```python
from build123d import *

# Parameters (mm, degrees)
F0_R     = 20.2565
F0_R_2   = 1.5875
F1_DEPTH = 1.27


with BuildPart() as f1:
    # F0 (on Top) → F1 (new body)
    with BuildSketch(Plane.XY):
        Circle(F0_R)
        with Locations((-11.1125, -11.1125)):
            Circle(F0_R_2, mode=Mode.SUBTRACT)
        with Locations((11.1125, -11.1125)):
            Circle(F0_R_2, mode=Mode.SUBTRACT)
        with Locations((-11.1125, 11.1125)):
            Circle(F0_R_2, mode=Mode.SUBTRACT)
        with BuildLine():
            ThreePointArc((0.317454, 9.341808), (6.720768, 6.496262), (9.3472, 0))
            ThreePointArc((9.3472, 0), (-6.496262, -6.720768), (-0.317454, 9.341808))
            ThreePointArc((-0.317454, 9.341808), (-0.002696, 9.664689), (0.3175, 9.3472))
            ThreePointArc((0.3175, 9.3472), (0.317489, 9.344504), (0.317454, 9.341808))
        make_face(mode=Mode.SUBTRACT)
        with Locations((11.1125, 11.1125)):
            Circle(F0_R_2, mode=Mode.SUBTRACT)
    extrude(amount=F1_DEPTH)


solid = f1.part
```
Read the model definition and answer for the solid it produces. Units are mm, in the model's axes. Coordinates: 2 decimals unless noted, no trailing zeros. Order: outer loops, then holes, each group sorted by start corner. A loop starts at its lowest first (then second) coordinate and runs counter-clockwise, first axis right, second up. Notation, with made-up numbers: (50.25, 40) - (106.25, 40) arc R16 cw to (106.25, 65) - close; hole circle Ø5 at (83, 71). An arc over 180 degrees is marked (long way). Answer as a JSON object with one key per item and string values. Group by question number.
Item 1: Section D-D (y = -15.5) is taken. Give the vertices of the cut face in (x, z).
Item 2: The mould has two halves that part along Y. Classify faces 1 (the face through (12.63, -10.64, 0.63)), 2 (the face through (-4.391, -19.775, 0.626)), 3 (the face through (9, -4, 1.27)): +Y half, -Y half, draft (parallel to the pull), parting line (faces both ways), or undercut.
Item 3: Consider probe 1 along Y at (x, z) = (0, 0.5); probe 2 along Y at (x, z) = (12.5, 0.25); probe 3 along Y at (x, z) = (-10, 1). Determine where each line is inside the solid, lowest interval first. Write a range as from..to.
Item 4: Section C-C (y = 3) is taken. Give the vertices of the cut face in (x, z).
Item 5: Flat-ended cylindrical pins translate along their axes: P1, Ø5, axis at x = 11.11, y = 11.11, coming from the -Z side; P2, Ø3, axis at x = 11.11, y = -11.11, coming from the +Z side. Find the tip coordinate at first contact, or state that the pin passes through.
Item 6: Section A-A (z = 0.4) is taken. State how many separate pieces and enclosed holes the cut face has, plus the area to 3 significant figures.
Item 7: Section B-B (x = -7.5) is taken. Give the vertices of the cut face in (y, z), plus the area to 3 significant figures.
Results are:
{
 "1": {"outline": "(-13.04, 0) - (13.04, 0) - (13.04, 1.27) - (-13.04, 1.27) - close"},
 "2": {"face 1": "undercut", "face 2": "parting line", "face 3": "draft"},
 "3": {"probe 1": "y = -20.26..-9.35, 9.66..20.26", "probe 2": "y = -15.94..-11.88, -10.34..10.34, 11.88..15.94", "probe 3": "y = -17.62..-12.24, -9.98..9.98, 12.24..17.62"},
 "4": {"outline": "(-20.03, 0) - (-8.85, 0) - (-8.85, 1.27) - (-20.03, 1.27) - close; (8.85, 0) - (20.03, 0) - (20.03, 1.27) - (8.85, 1.27) - close"},
 "5": {"P1": "stops at z = 0", "P2": "passes through"},
 "6": {"separate pieces": "1", "enclosed holes": "5", "area": "983 mm^2"},
 "7": {"outline": "(-18.82, 0) - (-5.58, 0) - (-5.58, 1.27) - (-18.82, 1.27) - close; (5.58, 0) - (18.82, 0) - (18.82, 1.27) - (5.58, 1.27) - close", "area": "33.6 mm^2"}
}
